Read the model definition and answer for the solid it produces. Units are mm, in the model's axes. Face numbers are marked on the shaded views. Give positions to 0.01 mm unless a question says otherwise; leave off trailing zeros. Order: outer loops, then holes, each group sorted by start corner. A loop starts at its lowest first (then second) coordinate and runs counter-clockwise, first axis right, second up. Notation, with made-up numbers: (-22.5, 49.25) - (-12.5, 49.25) arc R18 cw to (-12.5, 68.25) - close; hole circle Ø9 at (26, 22.5). An arc over 180 degrees is marked (long way). Return JSON: item names as keys, results as strings.
```python
from build123d import *

# Parameters (mm, degrees)
ESQUISSE1_W             = 14
ESQUISSE1_H             = 14
EXTRUSION1_DEPTH        = 14
CHANFREIN1_SIZE         = 14
ESQUISSE2_R             = 1
ENL_V_MAT_EXTRU_1_DEPTH = 25.248711306


with BuildPart() as part:
    # Esquisse1 → Extrusion1 (new body)
    with BuildSketch(Plane.XY):
        with Locations((7, 7)):
            Rectangle(ESQUISSE1_W, ESQUISSE1_H)
    extrude(amount=EXTRUSION1_DEPTH)

    # Chanfrein1
    chanfrein1_edges = [part.edges().sort_by_distance(p)[0] for p in [
        (7, 14, 14),
    ]]
    chamfer(chanfrein1_edges, length=CHANFREIN1_SIZE - 0.0001)  # a hair under: the kernel refuses the full size

    # Esquisse2 → Enlèv. mat.-Extru.1 (cut, through all)
    with BuildSketch(Plane.XZ):
        with Locations(Location((7, 7, 0), (0, 0, 270))):
            Circle(ESQUISSE2_R)
    extrude(amount=-ENL_V_MAT_EXTRU_1_DEPTH, mode=Mode.SUBTRACT)


solid = part.part
```
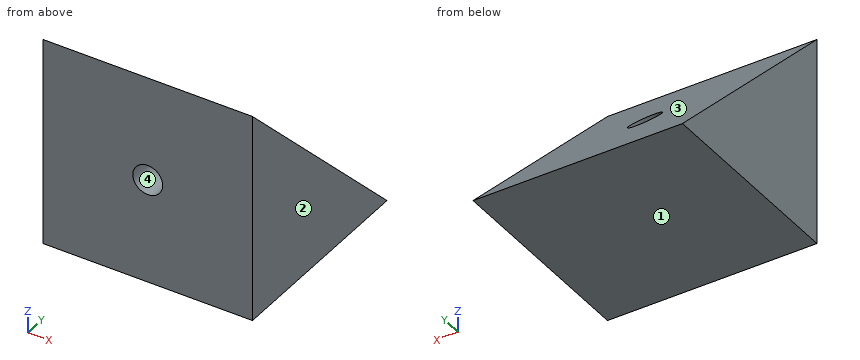
Q1. Determine the mould class of the marked faces 1, 2, 3 and 4 for opening direction Z: released by +Z, released by -Z, zero draft, split by the parting line, or undercut.
Values:
{"face 1": "released by -Z", "face 2": "zero draft", "face 3": "released by +Z", "face 4": "undercut"}
Q2. Given pin 1 (1.8 mm diameter, centred on x = 7, z = 7, fed in from -Y); pin 2 (1 mm diameter, centred on x = 10.5, y = 5, fed in from +Z); pin 3 (2 mm diameter, centred on x = 3, y = 10.5, fed in from +Z); pin 4 (1.5 mm diameter, centred on x = 2.5, y = 9, fed in from -Z), each flat-ended and moving along its own axis, determine where each tip first touches the part or whether it passes through.
Values:
{"pin 1": "passes through", "pin 2": "stops at z = 9.5", "pin 3": "stops at z = 4.5", "pin 4": "stops at z = 0"}
Q3. Consider L1, parallel to X at y = 5, z = 7; L2, parallel to Z at x = 12.75, y = 8; L3, parallel to Z at x = 7, y = 4.5. Determine where each line is inside the solid, lowest interval first.
Values:
{"L1": "x = 0 to 6, 8 to 14", "L2": "z = 0 to 6", "L3": "z = 0 to 6, 8 to 9.5"}
Q4. A cutting plane is placed at A-A (z = 7). Write down the section's boundary in (x, y).
Values:
{"outline": "(0, 0) - (6, 0) - (6, 7) - (0, 7) - close; (8, 0) - (14, 0) - (14, 7) - (8, 7) - close"}
Q5. A cutting plane is placed at D-D (y = 7.5). Write down the section's boundary in (x, z).
Values:
{"outline": "(0, 0) - (14, 0) - (14, 6.5) - (7.87, 6.5) arc R1 cw to (6.13, 6.5) - (0, 6.5) - close"}
